```python
from build123d import *

# Parameters (mm, degrees)
SKETCH001_R  = 1.5
POCKET_DEPTH = 2.001


with BuildPart() as part:
    # Sketch → Revolution (revolve)
    with BuildSketch(Plane.XZ):
        Polygon((-6.05, 0), (-24.05, 0), (-24.05, 2), (-9.05, 2), (-9.05, 28), (-11.05, 28), (-11.05, 30), (-6.05, 30), (-6.05, 27), (-7.55, 27), (-7.55, 25), (-6.05, 25), (-6.05, 4), (-7.55, 4), (-7.55, 2), (-6.05, 2), align=None)
    revolve(axis=Axis((0, 0, 0), (0, 0, 1)))

    # Sketch001 (on Face3 of Revolution) → Pocket (cut, through all)
    with BuildSketch(Plane(origin=(0, 0, 2), x_dir=(-1, 0, 0), z_dir=(0, 0, 1))):
        with Locations((0, 16)):
            Circle(SKETCH001_R)
        with Locations((0, -16)):
            Circle(SKETCH001_R)
        with Locations((16, 0)):
            Circle(SKETCH001_R)
        with Locations((-16, 0)):
            Circle(SKETCH001_R)
    extrude(amount=-POCKET_DEPTH, mode=Mode.SUBTRACT)


solid = part.part
```
Verification items for the finished model (mm, model axes). A direction names the side the tool comes from. Give positions to 0.01 mm unless a question says otherwise; leave off trailing zeros. Loops run counter-clockwise (first coordinate to the right, second up) from the corner with the lowest first, then second, coordinate; pieces in that order, holes last. Notation, with made-up numbers: M 34.5,-24.5 L 78.5,-24.5 A17 ccw 78.5,-14.5 Z; hole C -10,48.25 d1. An arc over 180 degrees is marked long. Return JSON: item names as keys, results as strings.
1) Gauge pin test, flat ends, axial feed: P1, Ø4, axis at x = 0, y = 16, coming from the -Z side; P2, Ø2, axis at x = -4, z = 5, coming from the -Y side; P3, Ø4, axis at x = 16, y = 0, coming from the +Z side. Record the tip position at first contact, or that the pin passes through.
Findings:
{"P1": "stops at z = 0", "P2": "stops at y = -8.54", "P3": "stops at z = 2"}
2) Material ranges on L1, parallel to Z at x = -6, y = -2; L2, parallel to Y at x = 0, z = 1.35; L3, parallel to Z at x = -9, y = -2.5, recorded low to high. Write a range as [from, to].
Findings:
{"L1": "z = [0, 2], [4, 25], [27, 30]", "L2": "y = [-24.05, -17.5], [-14.5, -6.05], [6.05, 14.5], [17.5, 24.05]", "L3": "z = [0, 2], [28, 30]"}
3) Mould release check, pull along Y, two halves, no side actions. Record for faces 1 (the flat face through (-5, 5, 30)), 2 (the cylindrical face through (-14.5, -0.07, 1.01)), 3 (the cylindrical face through (2.395, 10.787, 29.014)): released by +Y, released by -Y, zero draft, split by the parting line, or undercut.
Findings:
{"face 1": "zero draft", "face 2": "undercut", "face 3": "split by the parting line"}
4) Section check D-D, the plane x = -16. Enter the section's corners in (y, z), and give its area (3 significant figures).
Findings:
{"outline": "M -17.96,0 L -1.5,0 L -1.5,2 L -17.96,2 Z; M 1.5,0 L 17.96,0 L 17.96,2 L 1.5,2 Z", "area": "65.8 mm2"}
5) Section check C-C, the plane z = 7. Enter the section's corners in (x, y), and give its area (3 significant figures).
Findings:
{"outline": "C 0,0 d18.1; hole C 0,0 d12.1", "area": "142 mm2"}
6) Tool access check on faces 4 (the cylindrical face through (-5.589, 2.317, 0.986)), 5 (the cylindrical face through (1.64, 7.37, 2.99)). Record the directions out of +Z, -Z, +X, -X, +Y, -Y that give a thin tool (end or side, any length) a straight path to the whole face; none if there is none.
Findings:
{"face 4": "+Z, -Z", "face 5": "none"}
